Can you work these out from the drawing? Everything is in mm from the part's minimum corner. Coordinates: 2 decimals unless noted, no trailing zeros. Write each loop counter-clockwise with the first axis right and the second up, starting at its lowest first coordinate (ties: lowest second). Pieces come first, ordered by that corner, then holes.
(1) Imagine slicing it at D-D, the plane y = 39. List the corners of the cut face in (x, z) for me, plus the area to 3 significant figures.
(2) Imagine slicing it at B-B, the plane x = 25. List the corners of the cut face in (y, z) for me.
(3) Imagine slicing it at A-A, the plane y = 23. List the corners of the cut face in (x, z) for me.
(4) Please list where these lines run through material, in increasing order: probe 1 along X at (y, z) = (43, 5.5); probe 2 along Y at (x, z) = (30, 6.5); probe 3 along X at (y, z) = (74.5, 1.25).
(5) Thinking about a two-plate mould opening in Y: for the marked faces 1, 2, 3 and 4, which applies, released by +Y, released by -Y, zero draft, split by the parting line, or undercut?
(6) Imagine slicing it at C-C, the plane z = 3. List the corners of the cut face in (x, y) for me.
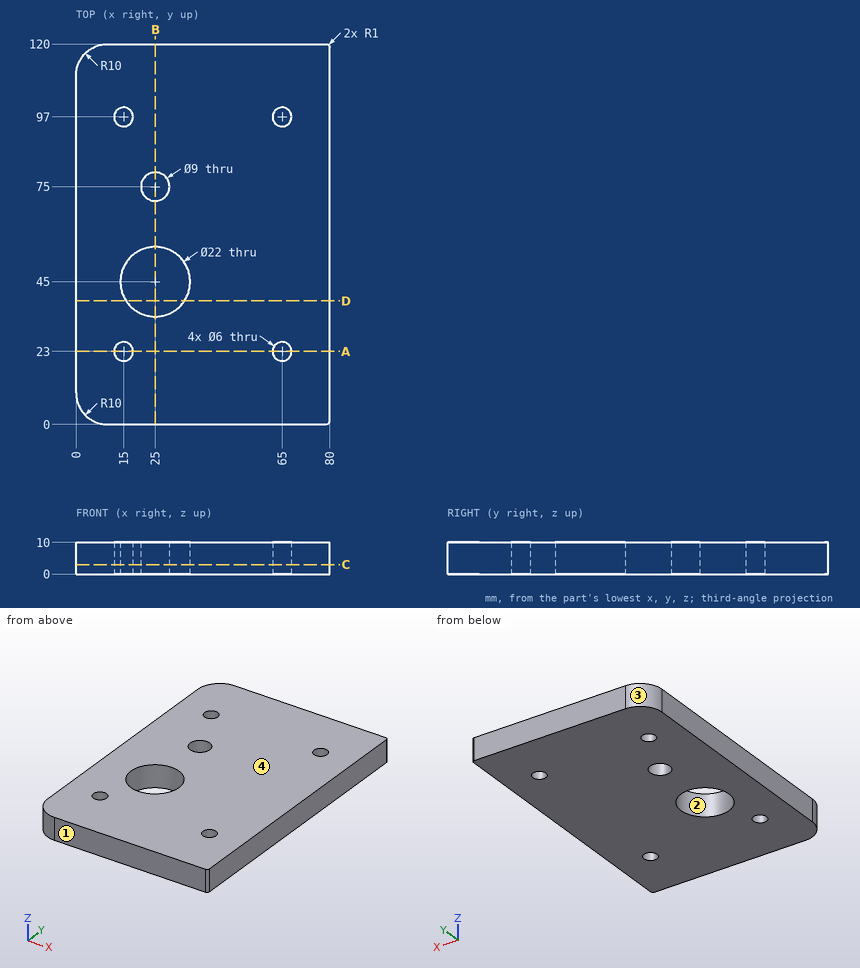
Recorded:
1. outline: (0, 0) - (15.78, 0) - (15.78, 10) - (0, 10) - close; (34.22, 0) - (80, 0) - (80, 10) - (34.22, 10) - close
1. area: 616 mm2
2. outline: (0, 0) - (34, 0) - (34, 10) - (0, 10) - close; (56, 0) - (70.5, 0) - (70.5, 10) - (56, 10) - close; (79.5, 0) - (120, 0) - (120, 10) - (79.5, 10) - close
3. outline: (0, 0) - (12, 0) - (12, 10) - (0, 10) - close; (18, 0) - (62, 0) - (62, 10) - (18, 10) - close; (68, 0) - (80, 0) - (80, 10) - (68, 10) - close
4. probe 1: x = 0 to 14.18, 35.82 to 80
4. probe 2: y = 0 to 35.2, 54.8 to 120
4. probe 3: x = 0 to 20.53, 29.47 to 80
5. face 1: released by -Y
5. face 2: undercut
5. face 3: released by +Y
5. face 4: zero draft
6. outline: (0, 10) arc R10 ccw to (10, 0) - (79, 0) arc R1 ccw to (80, 1) - (80, 119) arc R1 ccw to (79, 120) - (10, 120) arc R10 ccw to (0, 110) - close; hole circle Ø6 at (15, 23); hole circle Ø6 at (15, 97); hole circle Ø22 at (25, 45); hole circle Ø9 at (25, 75); hole circle Ø6 at (65, 23); hole circle Ø6 at (65, 97)
